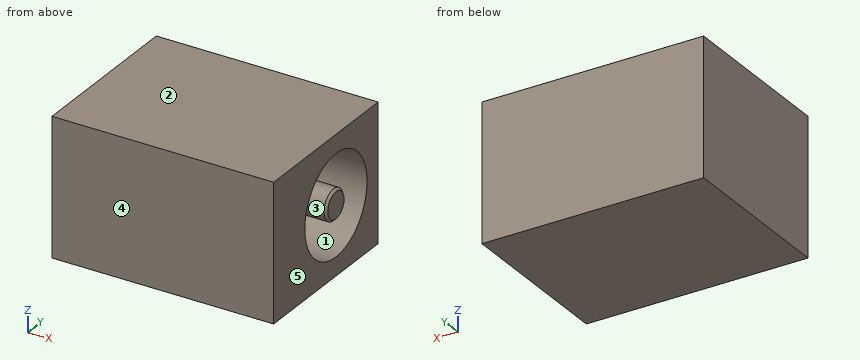
Autodesk Inventor part; units mm, degrees
ref_plane "YZ Plane" through (0, 0, 0) normal (1, 0, 0) x (0, 1, 0)
ref_plane "XZ Plane" through (0, 0, 0) normal (0, 1, 0) x (-1, 0, 0)
ref_plane "XY Plane" through (0, 0, 0) normal (0, 0, 1) x (1, 0, 0)
sketch "Szkic1" plane through (0, 0, 0) normal (0, 1, 0) x (-1, 0, 0)
  line L0 (14.4, -8.9) -> (0, -8.9)
  line L1 (0, -8.9) -> (0, 0)
  line L2 (0, 0) -> (14.4, 0)
  line L3 (14.4, 0) -> (14.4, -8.9)
  dimension "d0" = 8.9
  dimension "d1" = 14.4
extrude "Wyciągnięcie proste1" add sketch "Szkic1" along normal blind 10.9
sketch "Szkic2" plane through (0, 0, 0) normal (1, 0, 0) x (0, 0, -1)
  line L0 (0, 10.9) -> (8.9, 10.9)
  line L1 (4.45, 10.9) -> (4.45, 0)
  line L2 (0, 0) -> (8.9, 0)
  circle A0 centre (4.45, 6.5) radius 1
  circle A1 centre (4.45, 6.5) radius 3.25
  dimension "d4" = 2
  dimension "d5" = 6.5
  dimension "d6" = 6.5
extrude "Wyciągnięcie proste2" cut sketch "Szkic2" against normal blind 7 contours A1 L1 A0 | L1 A0 A1
chamfer "Faza1" distance 0.15 angle 45 1 edges at (0, 6.5, -3.45)
equation "\"d0\" = input_a"
equation "\"d1\" = input_b"
equation "\"d2\" = input_wys"
equation "\"gniazdo_M2_glebokosc\" = 1.5"
equation "\"gniazdo_M2_D1\" = 4.5"
equation "\"gniazdo_M2_D2\" = 2.6"
equation "\"insert_D\" = 2.9"
equation "\"insert_glebokosc\" = 7"
equation "\"podstawa_wys\" = 2"
equation "\"podstawa_otwory_montazowe_poz_x\" = 4"
equation "\"podstawa_otwory_montazowe_poz_y\" = 4"
equation "\"podstawa_zaokraglenie\" = 3"
equation "\"obudowa_wys\" = 45"
equation "\"obudowa_grubosc\" = 2"
equation "\"obudowa_kontrolki_a\" = 38"
equation "\"obudowa_otwory_montazowe_poz_x\" = 4"
equation "\"obudowa_otwory_montazowe_poz_y\" = 4"
equation "\"obudowa_otwory_montazowe_material_x\" = 8"
equation "\"obudowa_otwory_montazowe_material_y\" = 8"
equation "\"obudowa_zaokraglenie\" = 3"
equation "\"obudowa_otwory_io1_D\" = 12"
equation "\"obudowa_otwory_io1_wys\" = 25"
equation "\"obudowa_otwory_io1_poz\" = 55"
equation "\"obudowa_otwory_io2_D\" = 12"
equation "\"obudowa_otwory_io2_wys\" = 25"
equation "\"obudowa_otwory_io2_poz\" = 38"
equation "\"obudowa_otwory_pot_D\" = 7.2"
equation "\"input_a\" = 8.9"
equation "\"input_b\" = 14.4"
equation "\"input_wys\" = 10.9"
equation "\"obudowa_MTS_otwor_D\" = 6.2"
equation "\"obudowa_pot_poz_y\" = 15"
equation "\"obudowa_s_poz_x\" = 78"
equation "\"obudowa_s_D\" = 6.2"
equation "\"obudowa_s_poz_y\" = 15"
equation "\"obudowa_s_rozstaw_y\" = 16"
equation "\"pcb_rozstaw_x\" = 92"
equation "\"pcb_rozstaw_y\" = 58"
equation "\"obudowa_pcb_grubosc_scianki\" = 6"
equation "\"pcb_grubosc_scianki\" = 6"
equation "\"pcb_poz_y\" = 29"
equation "\"pcb_wys_bloku\" = 35"
equation "\"obudowa_footswitch_poz_y\" = 68"
equation "\"obudowa_footswitch_poz_x\" = 35"
equation "\"obudowa_footswitch_D\" = 12.3"
equation "\"obudowa_led_indicator_D\" = 3.5"
equation "\"obudowa_led_indicator_poz_x\" = 55"
equation "\"obudowa_podkladka_otwory\" = 4"
equation "\"podstawa_uchwyt_grubosc\" = 3"
equation "\"podstawa_uchwyt_wysokosc\" = 15"
equation "\"obudowa_uchwyt_grubosc\" = 2"
equation "\"pbudowa_uchwyt_podciecie_wys\" = 1.5"
equation "\"obudowa_uchwyt_wysokosc_wew\" = 26.3"
equation "\"obudowa_uchwyt_szerokosc_wew\" = 17.5"
equation "\"obudowa_gniazdo_poz\" = 25"
equation "\"obudowa_uchwyt_kolnierz_wys\" = 55"
equation "\"obudowa_uchwyt_poz_y\" = 2"
equation "\"obudowa_uchwyt_poz_z\" = 3"
equation "\"obudowa_podciecie_inout_wys\" = 6"
equation "\"obudowa_podciecie_logo_wys\" = 34"
equation "\"obudowa_podciecie_logo_szerokosc\" = 25"
equation "\"obudowa_pot_pozycjonowanie_wys\" = 13"
equation "\"obudowa_pot_pozycjonowanie_szerokosc\" = 2.8"
equation "\"obudowa_pot_pozycjonowanie_glebokosc\" = 1.4"
equation "\"obudowa_led_mocowanie_wys\" = 6"
equation "\"obudowa_led_mocowanie_poz\" = 46"
equation "\"obudowa_led_mocowanie_D\" = 5.5"
equation "\"obudowa_led_mocowanie_grubosc\" = 8"
equation "\"holder_led_grubosc\" = 2.5"
equation "\"holder_led_dlugosc\" = 28"
equation "\"holder_led_uchwyt_D\" = 5"
equation "\"holder_led_uchwyt_wysokosc\" = 5"
equation "\"holder_led_uchwyt_szerokosc\" = 8"
equation "\"holder_gniazdo_b\" = 5"
equation "\"holder_gniazdo_grubosc\" = 2.5"
equation "\"holder_gniazdo_a\" = 28"
equation "\"podstawa_mocowanie_DC_a\" = 7"
equation "\"podstawa_mocowanie_DC_b\" = 8.9"
equation "\"podstawa_mocowanie_DC_wys\" = 6"
equation "\"holder_gniazdo_odleglosc_miedzy_ramionami\" = 9.2"
equation "\"holder_gniazdo_grubosc_ramion\" = 1.5"
equation "\"holder_gniazdo_wys\" = 8"
equation "\"holder_gniazdo_uchwyt_poz\" = 5"
properties part number "9V_input" material "Polipropylen"
Design review of the part built by this model. Coordinates are the model's own, in mm. Face numbers are marked on the shaded views. A direction names the side the tool comes from. Coordinates: 2 decimals unless noted, no trailing zeros. Loops run counter-clockwise (first coordinate to the right, second up) from the corner with the lowest first, then second, coordinate; pieces in that order, holes last. Notation, with made-up numbers: (4.5, 62) -> (21.5, 62) arc R20 cw to (21.5, 73) -> close; hole circle Ø8 at (76.25, 45.5). An arc over 180 degrees is marked (long way). Use a Markdown table: item, result. Add a question column.
Item 1: We need section A-A, the plane y = 6.5. Write out the cut boundary in (x, z).
Item 2: The part is to be moulded in two halves that separate along Y. For the marked faces 3, 4 and 5, say which applies: +Y half, -Y half, draft (parallel to the pull), parting line (faces both ways), or undercut.
Item 3: Wall thickness on L1, parallel to Z at x = -2.75, y = 6.5; L2, parallel to Y at x = -2.75, z = -4.45; L3, parallel to Z at x = -3.25, y = 6: over which ranges is each line inside the solid? List them lowest first. Write a range as from..to.
Item 4: Machinability: for the marked faces 1 and 2, which of the approach directions +Z, -Z, +X, -X, +Y, -Y give a long, thin tool a straight path to every point of the face, cutting with its end or side? Answer none if there is none.
Item 5: We need section B-B, the plane z = -4.45. Write out the cut boundary in (x, y), and give its area (3 significant figures).
Item 6: Clearance check with a flat-ended pin moving along its axis: P1, Ø2, axis at y = 4.5, z = -3.5, coming from the +X side. State where the tip first meets the part, or that it passes through.
Item 7: We need section D-D, the plane y = 4.5. Write out the cut boundary in (x, z), and give its area (3 significant figures).
Item 8: We need section C-C, the plane z = -2. Write out the cut boundary in (x, y).
Numbers:
| question | item | result |
|---|---|---|
| 1 | outline | (-14.4, -8.9) -> (0, -8.9) -> (0, -7.7) -> (-7, -7.7) -> (-7, -5.45) -> (-0.15, -5.45) -> (0, -5.3) -> (0, -3.6) -> (-0.15, -3.45) -> (-7, -3.45) -> (-7, -1.2) -> (0, -1.2) -> (0, 0) -> (-14.4, 0) -> close |
| 2 | face 3 | undercut |
| 2 | face 4 | -Y half |
| 2 | face 5 | draft |
| 3 | L1 | z = -8.9..-7.7, -5.45..-3.45, -1.2..0 |
| 3 | L2 | y = 0..3.25, 5.5..7.5, 9.75..10.9 |
| 3 | L3 | z = -8.9..-7.66, -5.32..-3.58, -1.24..0 |
| 4 | face 1 | +X |
| 4 | face 2 | +Z, +X, -X, +Y, -Y |
| 5 | outline | (-14.4, 0) -> (0, 0) -> (0, 3.25) -> (-7, 3.25) -> (-7, 5.5) -> (-0.15, 5.5) -> (0, 5.65) -> (0, 7.35) -> (-0.15, 7.5) -> (-7, 7.5) -> (-7, 9.75) -> (0, 9.75) -> (0, 10.9) -> (-14.4, 10.9) -> close |
| 5 | area | 125 mm^2 |
| 6 | P1 | stops at x = -7 |
| 7 | outline | (-14.4, -8.9) -> (0, -8.9) -> (0, -7.01) -> (-7, -7.01) -> (-7, -1.89) -> (0, -1.89) -> (0, 0) -> (-14.4, 0) -> close |
| 7 | area | 92.3 mm^2 |
| 8 | outline | (-14.4, 0) -> (0, 0) -> (0, 4.36) -> (-7, 4.36) -> (-7, 8.64) -> (0, 8.64) -> (0, 10.9) -> (-14.4, 10.9) -> close |
